Autodesk Inventor part; units mm, degrees
ref_plane "Work Plane1" through (0, 0, -149) normal (0, 0, 1) x (1, 0, 0)
ref_plane "YZ Plane" through (0, 0, 0) normal (1, 0, 0) x (0, 1, 0)
ref_plane "XZ Plane" through (0, 0, 0) normal (0, 1, 0) x (-1, 0, 0)
sketch "Sketch1" plane through (0, 0, 0) normal (1, 0, 0) x (0, 1, 0)
  circle A0 centre (0, 0) radius 25
  arc A1 (-25, -19.1099) -> (25, -19.1099) centre (0, 31) ccw
  line L0 (0, 31) -> (0, 0) construction
  circle A2 centre (0, 0) radius 149 construction
  line L1 (-25, 0) -> (-25, -149)
  line L2 (-25, -149) -> (25, -149)
  line L3 (25, -149) -> (25, 0)
  line L4 (-25, -149) -> (-40, -149)
  line L5 (-40, -149) -> (-40, -143.5305)
  arc A3 (-40, -143.5305) -> (0, -149) centre (0, 0) ccw
  line L6 (0, 0) -> (0, -149)
  line L7 (-25, 0) -> (25, 0)
  point P0 (0, -25)
  point P1 (-25, -146.8877)
  dimension "d2" = 298
  dimension "d0" = 50
  dimension "d1" = 112
  dimension "d3" = 40
sketch "Sketch2" plane through (0, 0, 0) normal (0, 0, 1) x (1, 0, 0)
  circle A0 centre (0, 0) radius 10
  dimension "d7" = 20
revolve "Revolution1" add sketch "Sketch1" angle 360 about axis through (0, 0, 0) along (0, 0, -1) picked at (-1.8543, -16.4577) contours L7 L6 A0 | A0 A1 L1 | L6 A3 L1 A1
extrude "Extrusion1" cut sketch "Sketch1" against normal through all both and the other way through all contours L7 A0 | L3 A1 A0 | A0 L6 L7 | L7 L6 A0 | A0 A1 L1
ref_plane "Work Plane1" through (0, 0, -149) normal (0, 0, 1) x (1, 0, 0)
extrude "Extrusion2" cut sketch "Sketch2" along normal blind 70 from surface at -149
fillet "Fillet1" radius 8 1 edges at (0, 25, -146.8877)
properties part number "shank"
For this review, take the finished solid that the model builds, in its own axes (mm). Give positions to 0.01 mm unless a question says otherwise; leave off trailing zeros. Order: outer loops, then holes, each group sorted by start corner. A loop starts at its lowest first (then second) coordinate and runs counter-clockwise, first axis right, second up. Notation, with made-up numbers: M -28,-3 L 28,-3 A10 ccw 28,5 Z; hole C 12,76 d2. An arc over 180 degrees is marked long. Answer in a Markdown table with one row per item. Add a question column.
(1) Mouldability with a two-part tool opening along X and no side actions: class faces 1 (the face through (-7.509, -23.846, -80.386)), 2 (the face through (0, 0, -25)), 3 (the face through (-2.17, 9.76, -114.32)) as +X half, -X half, draft (parallel to the pull), parting line (faces both ways), or undercut.
(2) Wall thickness on probe 1 along Y at (x, z) = (0, -121); probe 2 along Y at (x, z) = (4, -80): over which ranges is each line inside the solid? List them lowest first. Write a range as [from, to].
(3) Consider section A-A on z = -135. State the section outline as (x, y) points, and give its area (3 significant figures).
(4) For pin 1 (10 mm diameter, centred on y = -6, z = -114.5, fed in from +X); pin 2 (6 mm diameter, centred on y = -13.5, z = -127, fed in from -X); pin 3 (1.5 mm diameter, centred on x = -4.5, y = -12.5, fed in from +Z), all flat-tipped, find the tip position at first contact; note any pin that passes through.
Evaluation:
| question | item | result |
|---|---|---|
| 1 | face 1 | parting line |
| 1 | face 2 | draft |
| 1 | face 3 | undercut |
| 2 | probe 1 | y = [-25, -10], [10, 25] |
| 2 | probe 2 | y = [-24.68, -9.17], [9.17, 24.68] |
| 3 | outline | C 0,0 d50; hole C 0,0 d20 |
| 3 | area | 1,650 mm^2 |
| 4 | pin 1 | stops at x = 24.98 |
| 4 | pin 2 | stops at x = -22.69 |
| 4 | pin 3 | stops at z = -23.41 |
